from build123d import *

# Parameters (mm, degrees)
SKETCH_1_R      = 3.399999997
EXTRUDE_1_DEPTH = 50


with BuildPart() as part:
    # 草图1 → 凸台-拉伸1 (new, symmetric)
    with BuildSketch(Plane.XY):
        with BuildLine():
            Line((12.49999999, 14.999999989), (-12.49999999, 14.999999989))
            ThreePointArc((-12.49999999, 14.999999989), (-14.267766942, 14.267766942), (-14.999999989, 12.49999999))
            Line((-14.999999989, 12.49999999), (-14.999999989, -12.49999999))
            ThreePointArc((-14.999999989, -12.49999999), (-14.267766942, -14.267766942), (-12.49999999, -14.999999989))
            Line((-12.49999999, -14.999999989), (-5.399999996, -14.999999989))
            ThreePointArc((-5.399999996, -14.999999989), (-5.187867962, -14.912132023), (-5.099999996, -14.699999989))
            Line((-5.099999996, -14.699999989), (-5.099999996, -14.299999989))
            ThreePointArc((-5.099999996, -14.299999989), (-5.01213203, -14.087867955), (-4.799999996, -13.999999989))
            Line((-4.799999996, -13.999999989), (-4.399999997, -13.999999989))
            ThreePointArc((-4.399999997, -13.999999989), (-4.187867962, -13.912132024), (-4.099999997, -13.69999999))
            Line((-4.099999997, -13.69999999), (-4.099999997, -13.09999999))
            ThreePointArc((-4.099999997, -13.09999999), (-4.187867962, -12.887867956), (-4.399999997, -12.79999999))
            Line((-4.399999997, -12.79999999), (-7.949999994, -12.79999999))
            ThreePointArc((-7.949999994, -12.79999999), (-8.162132028, -12.712132025), (-8.249999994, -12.499999991))
            Line((-8.249999994, -12.499999991), (-8.249999994, -9.92989898))
            ThreePointArc((-8.249999994, -9.92989898), (-8.227163854, -9.81509395), (-8.162132028, -9.717766946))
            Line((-8.162132028, -9.717766946), (-4.332233044, -5.887867961))
            ThreePointArc((-4.332233044, -5.887867961), (-4.234906039, -5.822836136), (-4.12010101, -5.799999996))
            Line((-4.12010101, -5.799999996), (4.12010101, -5.799999996))
            ThreePointArc((4.12010101, -5.799999996), (4.234906039, -5.822836136), (4.332233044, -5.887867961))
            Line((4.332233044, -5.887867961), (8.162132028, -9.717766946))
            ThreePointArc((8.162132028, -9.717766946), (8.227163854, -9.81509395), (8.249999994, -9.92989898))
            Line((8.249999994, -9.92989898), (8.249999994, -12.499999991))
            ThreePointArc((8.249999994, -12.499999991), (8.162132028, -12.712132025), (7.949999994, -12.79999999))
            Line((7.949999994, -12.79999999), (4.399999997, -12.79999999))
            ThreePointArc((4.399999997, -12.79999999), (4.187867962, -12.887867956), (4.099999997, -13.09999999))
            Line((4.099999997, -13.09999999), (4.099999997, -13.69999999))
            ThreePointArc((4.099999997, -13.69999999), (4.187867962, -13.912132024), (4.399999997, -13.999999989))
            Line((4.399999997, -13.999999989), (4.799999996, -13.999999989))
            ThreePointArc((4.799999996, -13.999999989), (5.01213203, -14.087867955), (5.099999996, -14.299999989))
            Line((5.099999996, -14.299999989), (5.099999996, -14.699999989))
            ThreePointArc((5.099999996, -14.699999989), (5.187867962, -14.912132023), (5.399999996, -14.999999989))
            Line((5.399999996, -14.999999989), (12.49999999, -14.999999989))
            ThreePointArc((12.49999999, -14.999999989), (14.267766942, -14.267766942), (14.999999989, -12.49999999))
            Line((14.999999989, -12.49999999), (14.999999989, 12.49999999))
            ThreePointArc((14.999999989, 12.49999999), (14.267766942, 14.267766942), (12.49999999, 14.999999989))
        make_face()
        Circle(SKETCH_1_R, mode=Mode.SUBTRACT)
        with BuildLine():
            Line((7.949999994, 12.79999999), (-7.949999994, 12.79999999))
            ThreePointArc((-7.949999994, 12.79999999), (-8.162132028, 12.712132025), (-8.249999994, 12.499999991))
            Line((-8.249999994, 12.499999991), (-8.249999994, 9.92989898))
            ThreePointArc((-8.249999994, 9.92989898), (-8.227163854, 9.81509395), (-8.162132028, 9.717766946))
            Line((-8.162132028, 9.717766946), (-4.332233044, 5.887867961))
            ThreePointArc((-4.332233044, 5.887867961), (-4.234906039, 5.822836136), (-4.12010101, 5.799999996))
            Line((-4.12010101, 5.799999996), (4.12010101, 5.799999996))
            ThreePointArc((4.12010101, 5.799999996), (4.234906039, 5.822836136), (4.332233044, 5.887867961))
            Line((4.332233044, 5.887867961), (8.162132028, 9.717766946))
            ThreePointArc((8.162132028, 9.717766946), (8.227163853, 9.81509395), (8.249999994, 9.92989898))
            Line((8.249999994, 9.92989898), (8.249999994, 12.499999991))
            ThreePointArc((8.249999994, 12.499999991), (8.162132028, 12.712132025), (7.949999994, 12.79999999))
        make_face(mode=Mode.SUBTRACT)
        with BuildLine():
            Line((10.749999992, 9.749999993), (12.499999991, 9.749999993))
            ThreePointArc((12.499999991, 9.749999993), (13.207106771, 10.042893211), (13.49999999, 10.749999992))
            Line((13.49999999, 10.749999992), (13.49999999, 12.49999999))
            ThreePointArc((13.49999999, 12.49999999), (13.207106771, 13.207106771), (12.49999999, 13.49999999))
            Line((12.49999999, 13.49999999), (10.749999992, 13.49999999))
            ThreePointArc((10.749999992, 13.49999999), (10.042893211, 13.207106771), (9.749999993, 12.499999991))
            Line((9.749999993, 12.499999991), (9.749999993, 10.749999992))
            ThreePointArc((9.749999993, 10.749999992), (10.042893211, 10.042893211), (10.749999992, 9.749999993))
        make_face(mode=Mode.SUBTRACT)
        with BuildLine():
            Line((-13.49999999, 12.49999999), (-13.49999999, 10.749999992))
            ThreePointArc((-13.49999999, 10.749999992), (-13.207106771, 10.042893211), (-12.499999991, 9.749999993))
            Line((-12.499999991, 9.749999993), (-10.749999992, 9.749999993))
            ThreePointArc((-10.749999992, 9.749999993), (-10.042893211, 10.042893211), (-9.749999993, 10.749999992))
            Line((-9.749999993, 10.749999992), (-9.749999993, 12.499999991))
            ThreePointArc((-9.749999993, 12.499999991), (-10.042893211, 13.207106771), (-10.749999992, 13.49999999))
            Line((-10.749999992, 13.49999999), (-12.49999999, 13.49999999))
            ThreePointArc((-12.49999999, 13.49999999), (-13.207106771, 13.207106771), (-13.49999999, 12.49999999))
        make_face(mode=Mode.SUBTRACT)
        with BuildLine():
            Line((9.749999993, -10.749999992), (9.749999993, -12.499999991))
            ThreePointArc((9.749999993, -12.499999991), (10.042893211, -13.207106771), (10.749999992, -13.49999999))
            Line((10.749999992, -13.49999999), (12.49999999, -13.49999999))
            ThreePointArc((12.49999999, -13.49999999), (13.207106771, -13.207106771), (13.49999999, -12.49999999))
            Line((13.49999999, -12.49999999), (13.49999999, -10.749999992))
            ThreePointArc((13.49999999, -10.749999992), (13.207106771, -10.042893211), (12.499999991, -9.749999993))
            Line((12.499999991, -9.749999993), (10.749999992, -9.749999993))
            ThreePointArc((10.749999992, -9.749999993), (10.042893211, -10.042893211), (9.749999993, -10.749999992))
        make_face(mode=Mode.SUBTRACT)
        with BuildLine():
            Line((-5.799999996, -4.12010101), (-5.799999996, 4.12010101))
            ThreePointArc((-5.799999996, 4.12010101), (-5.822836136, 4.234906039), (-5.887867961, 4.332233044))
            Line((-5.887867961, 4.332233044), (-9.717766946, 8.162132028))
            ThreePointArc((-9.717766946, 8.162132028), (-9.81509395, 8.227163854), (-9.92989898, 8.249999994))
            Line((-9.92989898, 8.249999994), (-12.499999991, 8.249999994))
            ThreePointArc((-12.499999991, 8.249999994), (-12.712132025, 8.162132028), (-12.79999999, 7.949999994))
            Line((-12.79999999, 7.949999994), (-12.79999999, -7.949999994))
            ThreePointArc((-12.79999999, -7.949999994), (-12.712132025, -8.162132028), (-12.499999991, -8.249999994))
            Line((-12.499999991, -8.249999994), (-9.92989898, -8.249999994))
            ThreePointArc((-9.92989898, -8.249999994), (-9.81509395, -8.227163854), (-9.717766946, -8.162132028))
            Line((-9.717766946, -8.162132028), (-5.887867961, -4.332233044))
            ThreePointArc((-5.887867961, -4.332233044), (-5.822836136, -4.234906039), (-5.799999996, -4.12010101))
        make_face(mode=Mode.SUBTRACT)
        with BuildLine():
            Line((5.799999996, 4.12010101), (5.799999996, -4.12010101))
            ThreePointArc((5.799999996, -4.12010101), (5.822836136, -4.234906039), (5.887867961, -4.332233044))
            Line((5.887867961, -4.332233044), (9.717766946, -8.162132028))
            ThreePointArc((9.717766946, -8.162132028), (9.81509395, -8.227163854), (9.92989898, -8.249999994))
            Line((9.92989898, -8.249999994), (12.499999991, -8.249999994))
            ThreePointArc((12.499999991, -8.249999994), (12.712132025, -8.162132028), (12.79999999, -7.949999994))
            Line((12.79999999, -7.949999994), (12.79999999, 7.949999994))
            ThreePointArc((12.79999999, 7.949999994), (12.712132025, 8.162132028), (12.499999991, 8.249999994))
            Line((12.499999991, 8.249999994), (9.92989898, 8.249999994))
            ThreePointArc((9.92989898, 8.249999994), (9.81509395, 8.227163854), (9.717766946, 8.162132028))
            Line((9.717766946, 8.162132028), (5.887867961, 4.332233044))
            ThreePointArc((5.887867961, 4.332233044), (5.822836136, 4.234906039), (5.799999996, 4.12010101))
        make_face(mode=Mode.SUBTRACT)
        with BuildLine():
            Line((-10.749999992, -9.749999993), (-12.499999991, -9.749999993))
            ThreePointArc((-12.499999991, -9.749999993), (-13.207106771, -10.042893211), (-13.49999999, -10.749999992))
            Line((-13.49999999, -10.749999992), (-13.49999999, -12.49999999))
            ThreePointArc((-13.49999999, -12.49999999), (-13.207106771, -13.207106771), (-12.49999999, -13.49999999))
            Line((-12.49999999, -13.49999999), (-10.749999992, -13.49999999))
            ThreePointArc((-10.749999992, -13.49999999), (-10.042893211, -13.207106771), (-9.749999993, -12.499999991))
            Line((-9.749999993, -12.499999991), (-9.749999993, -10.749999992))
            ThreePointArc((-9.749999993, -10.749999992), (-10.042893211, -10.042893211), (-10.749999992, -9.749999993))
        make_face(mode=Mode.SUBTRACT)
    extrude(amount=EXTRUDE_1_DEPTH, both=True)


solid = part.part
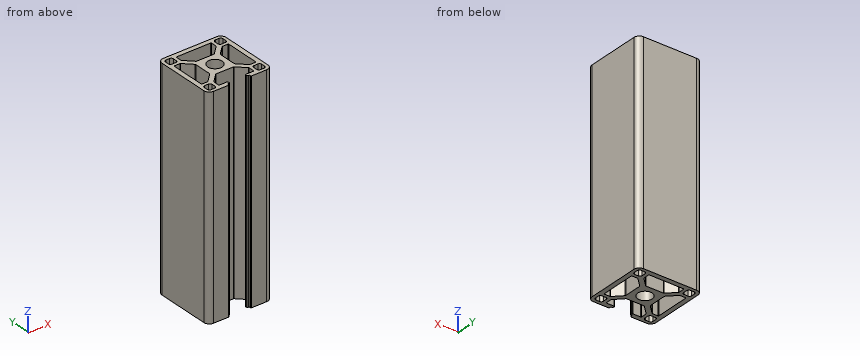
Geometry check sheet. Reference: the model listing, model coordinates, mm. Give positions to 0.01 mm unless a question says otherwise; leave off trailing zeros. Loops run counter-clockwise (first coordinate to the right, second up) from the corner with the lowest first, then second, coordinate; pieces in that order, holes last. Notation, with made-up numbers: (-14, 41) -> (39, 41) arc R29 cw to (39, 75) -> close; hole circle Ø5 at (50.25, 26.5). An arc over 180 degrees is marked (long way). Answer in a Markdown table with one row per item. Add a question column.
1) Gauge pin test, flat end, axial feed: P1, Ø0.5, axis at y = -13.5, z = -2, coming from the -X side. Record the tip position at first contact, or that the pin passes through.
2) Cross-section at C-C on z = -19. State how many separate pieces and enclosed holes the cut face has, and give its area (3 significant figures).
3) Cross-section at A-A on x = 0. Record the boundary of the cut face in (y, z).
4) Material ranges on probe 1 along X at (y, z) = (-11.5, -40.5); probe 2 along Y at (x, z) = (0, 3.5), recorded low to high. Write a range as from..to.
5) Cross-section at B-B on y = 0. Record the boundary of the cut face in (x, z), and give its area (3 significant figures).
Outcome:
| question | item | result |
|---|---|---|
| 1 | P1 | stops at x = -14.88 |
| 2 | separate pieces | 1 |
| 2 | enclosed holes | 8 |
| 2 | area | 388 mm^2 |
| 3 | outline | (-5.8, -50) -> (-3.4, -50) -> (-3.4, 50) -> (-5.8, 50) -> close; (3.4, -50) -> (5.8, -50) -> (5.8, 50) -> (3.4, 50) -> close; (12.8, -50) -> (15, -50) -> (15, 50) -> (12.8, 50) -> close |
| 4 | probe 1 | x = -15..-13.5, -9.75..-8.25, 8.25..9.75, 13.5..15 |
| 4 | probe 2 | y = -5.8..-3.4, 3.4..5.8, 12.8..15 |
| 5 | outline | (-15, -50) -> (-12.8, -50) -> (-12.8, 50) -> (-15, 50) -> close; (-5.8, -50) -> (-3.4, -50) -> (-3.4, 50) -> (-5.8, 50) -> close; (3.4, -50) -> (5.8, -50) -> (5.8, 50) -> (3.4, 50) -> close; (12.8, -50) -> (15, -50) -> (15, 50) -> (12.8, 50) -> close |
| 5 | area | 920 mm^2 |
